from build123d import *

# Parameters (mm, degrees)
BOSS_EXTRUDE1_DEPTH   = 144
CHAMFER1_SIZE         = 1.5
CHAMFER2_SIZE         = 3
F_6_32_TAPPED_HOLE1_D = 2.7051
F_6_CLEARANCE_HOLE1_D = 3.6576


with BuildPart() as part:
    # Sketch1 → Boss-Extrude1 (new body, symmetric)
    with BuildSketch(Plane(origin=(0, 0, 0), x_dir=(0, 0, -1), z_dir=(1, 0, 0))):
        Polygon((0, 0), (31.75, 0), (31.75, 3.175), (3.175, 3.175), (3.175, 31.75), (0, 31.75), align=None)
    extrude(amount=BOSS_EXTRUDE1_DEPTH, both=True)

    # Chamfer1
    chamfer1_edges = [part.edges().sort_by_distance(p)[0] for p in [
        (0, 31.75, -3.175),
        (0, 3.175, -3.175),
        (0, 3.175, -31.75),
    ]]
    chamfer(chamfer1_edges, length=CHAMFER1_SIZE)

    # Chamfer2
    chamfer2_edges = [part.edges().sort_by_distance(p)[0] for p in [
        (-144, 31.75, -0.8375),
        (-144, 0.8375, -31.75),
        (144, 0.8375, -31.75),
        (144, 31.75, -0.8375),
    ]]
    chamfer(chamfer2_edges, length=CHAMFER2_SIZE)

    # #6-32 Tapped Hole1 (through all)
    with Locations(Plane(origin=(0, 3.175, 0), x_dir=(1, 0, 0), z_dir=(0, 1, 0))):
        with Locations((-136, 27.221), (-120, 27.221), (-128, 19.221), (-136, 11.221), (-120, 11.221), (120, 27.221), (136, 27.221), (128, 19.221), (120, 11.221), (136, 11.221)):
            Hole(F_6_32_TAPPED_HOLE1_D / 2)

    # #6 Clearance Hole1 (through all)
    with Locations(Plane(origin=(0, 0, -3.175), x_dir=(-1, 0, 0), z_dir=(0, 0, -1))):
        with Locations((0, 24), (-8, 16), (8, 16), (0, 8), (24, 16), (32, 24), (40, 16), (32, 8)):
            Hole(F_6_CLEARANCE_HOLE1_D / 2)


solid = part.part
Geometry: final body of the model. Coordinates: model frame, mm. A direction names the side the tool comes from. Give positions to 0.01 mm unless a question says otherwise; leave off trailing zeros. Loops run counter-clockwise (first coordinate to the right, second up) from the corner with the lowest first, then second, coordinate; pieces in that order, holes last. Notation, with made-up numbers: (-10.5, 14) - (6.5, 14) arc R21 cw to (6.5, 38) - close; hole circle Ø6 at (7.5, -18). An arc over 180 degrees is marked (long way). Answer as CSV lines item,"result". Start each with the question number.
1. Section A-A, the plane x = -69.5. Return loops of the section in (y, z) (3 decimals), plus the area to 3 significant figures.
2. Ray query, L1, parallel to X at y = 3, z = -11.5; L2, parallel to Z at x = 136, y = 2.25 (3 decimals); L3, parallel to X at y = 16.5, z = -3. Return the intervals inside material, ascending.
3. Pin query (flat end, axial travel): P1, Ø4, axis at x = 21.5, y = 14.5, coming from the -Z side (3 decimals); P2, Ø2, axis at x = -136, z = -11.221, coming from the -Y side; P3, Ø4.5, axis at x = 136, z = -11.221, coming from the +Y side (3 decimals). Return the tip coordinate at first contact, or that it passes through.
4. Reachability of faces 1 (the face through (2, 17, -3.175)), 2 (the face through (144, 8, -3)) from +Z, -Z, +X, -X, +Y, -Y: full face, straight path, thin tool, end or side. Return the list, or none.
Answers:
1,outline,"(0, -31.75) - (1.675, -31.75) - (3.175, -30.25) - (3.175, -4.675) - (4.675, -3.175) - (30.25, -3.175) - (31.75, -1.675) - (31.75, 0) - (0, 0) - close"
1,area,"190 mm2"
2,L1,"x = -144 to -137.32, -134.68 to -121.32, -118.68 to 118.68, 121.32 to 134.68, 137.32 to 144"
2,L2,"z = -31.175 to -28.574, -25.868 to -12.574, -9.868 to 0"
2,L3,"x = -144 to -41.76, -38.24 to -25.76, -22.24 to -9.76, -6.24 to 6.24, 9.76 to 144"
3,P1,"stops at z = -3.175"
3,P2,"passes through"
3,P3,"stops at y = 3.175"
4,face 1,"-Z, +X, -X, +Y"
4,face 2,"+Z, -Z, +X, +Y, -Y"
